```python
from build123d import *

# Parameters (mm, degrees)
EXTRUSION1_DEPTH   = 6.35
HOLE1_D            = 6.35
EXTRUSION2_DEPTH   = 25.4
SKETCH5_W          = 38.1
SKETCH5_H          = 84.141733333
CUT_EXTRUDE1_DEPTH = 230.421522185


with BuildPart() as part:
    # Sketch1 → Extrusion1 (new body)
    with BuildSketch(Plane.XY):
        Polygon((-136.071428881, 83.003571429), (16.328571119, -18.596428571), (67.128571119, -18.596428571), (67.128571119, 184.603571429), (-136.071428881, 184.603571429), align=None)
    extrude(amount=EXTRUSION1_DEPTH)

    # Hole1 (through all)
    with Locations(Plane.XY.offset(6.35)):
        with Locations((-123.371428881, 171.903571429), (-97.971428881, 171.903571429), (-72.571428881, 171.903571429), (-47.171428881, 171.903571429), (-21.771428881, 171.903571429), (3.628571119, 171.903571429), (29.028571119, 171.903571429), (54.428571119, 171.903571429), (-123.371428881, 146.503571429), (-97.971428881, 146.503571429), (-72.571428881, 146.503571429), (-47.171428881, 146.503571429), (-21.771428881, 146.503571429), (3.628571119, 146.503571429), (29.028571119, 146.503571429), (54.428571119, 146.503571429), (-123.371428881, 121.103571429), (-97.971428881, 121.103571429), (-72.571428881, 121.103571429), (-47.171428881, 121.103571429), (-21.771428881, 121.103571429), (3.628571119, 121.103571429), (29.028571119, 121.103571429), (54.428571119, 121.103571429), (-123.371428881, 95.703571429), (-97.971428881, 95.703571429), (-72.571428881, 95.703571429), (-47.171428881, 95.703571429), (-21.771428881, 95.703571429), (3.628571119, 95.703571429), (29.028571119, 95.703571429), (54.428571119, 95.703571429), (54.428571119, 70.303571429), (54.428571119, 44.903571429), (54.428571119, 19.503571429), (54.428571119, -5.896428571), (29.028571119, 70.303571429), (29.028571119, 44.903571429), (29.028571119, 19.503571429), (29.028571119, -5.896428571)):
            Hole(HOLE1_D / 2)

    # Sketch4 → Extrusion2 (cut)
    with BuildSketch(Plane(origin=(0, 0, 0), x_dir=(-1, 0, 0), z_dir=(0, 0, -1))):
        Polygon((33.684028881, 65.545304762), (33.684028881, 14.745304762), (109.884028881, 65.545304762), align=None)
    extrude(amount=-EXTRUSION2_DEPTH, mode=Mode.SUBTRACT)

    # Sketch5 → Cut-Extrude1 (cut, through all)
    with BuildSketch(Plane.XY.offset(6.35)):
        with Locations((-14.634028881, 23.474438095)):
            Rectangle(SKETCH5_W, SKETCH5_H)
    extrude(amount=-CUT_EXTRUDE1_DEPTH, mode=Mode.SUBTRACT)


solid = part.part
```
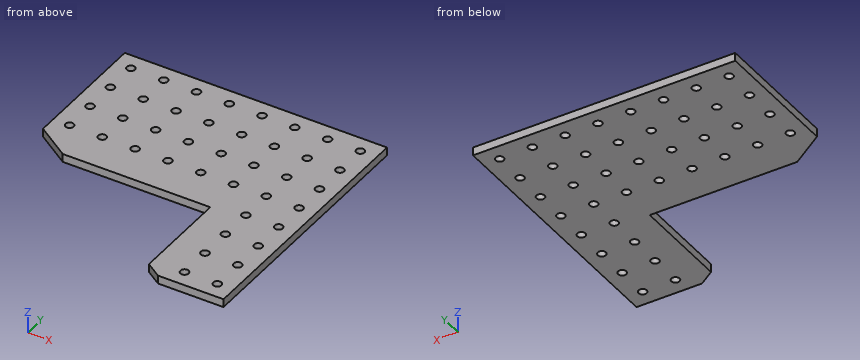
Could you check a few things on this model? Use its own coordinates, in mm. Coordinates: 2 decimals unless noted, no trailing zeros. Loops run counter-clockwise (first coordinate to the right, second up) from the corner with the lowest first, then second, coordinate; pieces in that order, holes last.
1) Please list where these lines run through material, in increasing order: line 1 along Y through (x, z) = (-121, 2.5); line 2 along X through (y, z) = (21.5, 6); line 3 along Y through (x, z) = (-88.5, 4.25).
Reported:
line 1: y = 72.96 to 93.59, 97.81 to 118.99, 123.21 to 144.39, 148.61 to 169.79, 174.01 to 184.6
line 2: x = 4.42 to 26.56, 31.5 to 51.96, 56.9 to 67.13
line 3: y = 65.55 to 184.6
2) Imagine slicing it at A-A (x = -21). List the corners of the cut face in (y, z) for me.
Reported:
outline: (65.55, 0) - (92.62, 0) - (92.62, 6.35) - (65.55, 6.35) - close; (98.78, 0) - (118.02, 0) - (118.02, 6.35) - (98.78, 6.35) - close; (124.18, 0) - (143.42, 0) - (143.42, 6.35) - (124.18, 6.35) - close; (149.58, 0) - (168.82, 0) - (168.82, 6.35) - (149.58, 6.35) - close; (174.98, 0) - (184.6, 0) - (184.6, 6.35) - (174.98, 6.35) - close
3) Will this pin go through, and if not, where does the flat tip stop? pin 1 Ø10 at (x, y) = (32.5, 150) entering from -Z.
Reported:
pin 1: stops at z = 0
4) Imagine slicing it at C-C (z = 2.75). State how many separate pieces and enclosed holes the cut face has, and give its area (3 significant figures).
Reported:
separate pieces: 1
enclosed holes: 40
area: 27,900 mm2
5) Imagine slicing it at D-D (y = 78). List the corners of the cut face in (x, z) for me, and give its area (3 significant figures).
Reported:
outline: (-128.57, 0) - (67.13, 0) - (67.13, 6.35) - (-128.57, 6.35) - close
area: 1,240 mm2
6) Imagine slicing it at B-B (y = 29.5). List the corners of the cut face in (x, z) for me, and give its area (3 significant figures).
Reported:
outline: (4.42, 0) - (67.13, 0) - (67.13, 6.35) - (4.42, 6.35) - close
area: 398 mm2
